Autodesk Inventor part; units mm, degrees
ref_plane "YZ Plane" through (0, 0, 0) normal (1, 0, 0) x (0, 1, 0)
ref_plane "XZ Plane" through (0, 0, 0) normal (0, 1, 0) x (-1, 0, 0)
ref_plane "XY Plane" through (0, 0, 0) normal (0, 0, 1) x (1, 0, 0)
sketch "Sketch1" plane through (0, 0, 0) normal (1, 0, 0) x (0, 1, 0)
  line L0 (0, 0) -> (25.4, 0)
  line L1 (25.4, 0) -> (25.4, -133.35)
  line L2 (25.4, -133.35) -> (0, -133.35)
  line L3 (0, -133.35) -> (0, 0)
  dimension "d0" = 25.4
  dimension "d1" = 133.35
extrude "Extrusion1" add sketch "Sketch1" along normal blind 6.35
sketch "Sketch2" plane through (6.35, 0, 0) normal (1, 0, 0) x (0, 0, -1)
  line L0 (133.35, 0) -> (133.35, 25.4)
  line L1 (133.35, 25.4) -> (0, 25.4)
  line L2 (0, 25.4) -> (0, 0)
  line L3 (0, 0) -> (133.35, 0)
  circle A0 centre (12.7, 12.7) radius 6.35
  circle A1 centre (120.65, 12.7) radius 6.35
  dimension "d4" = 25.4
  dimension "d5" = 12.7
  dimension "d6" = 12.7
  dimension "d7" = 107.95
  dimension "d8" = 133.35
  dimension "d9" = 12.7
  dimension "d10" = 12.7
  dimension "d11" = 12.7
extrude "Extrusion2" cut sketch "Sketch2" against normal blind 6.35 contours A0 | A1
sketch "Sketch3" plane through (6.35, 0, 0) normal (1, 0, 0) x (0, 0, -1)
  circle A0 centre (12.7, 12.7) radius 6.35
  circle A1 centre (12.7, 12.7) radius 12.7
  line L0 (133.35, 25.4) -> (0, 25.4)
  line L1 (0, 25.4) -> (0, 0)
  line L2 (0, 0) -> (133.35, 0)
  point P0 (12.7, 0)
  point P1 (0, 12.7)
  point P2 (12.7, 25.4)
extrude "Extrusion3" cut sketch "Sketch3" against normal blind 6.35 contours A1 L1 L0 | L2 L1 A1
sketch "Sketch4" plane through (6.35, 0, 0) normal (1, 0, 0) x (0, 0, -1)
  circle A0 centre (12.7, 12.7) radius 6.35
  line L0 (120.65, 12.7) -> (12.7, 12.7)
  circle A1 centre (120.65, 12.7) radius 6.35
  line L1 (12.7, 12.7) -> (120.65, -43.3755)
  line L2 (120.65, -43.3755) -> (120.65, 12.7)
  line L3 (12.7, 12.7) -> (9.1874, 5.9379)
  line L4 (9.1874, 5.9379) -> (43.1586, -11.7087)
  line L5 (43.1586, -11.7087) -> (46.6713, -4.9467)
  line L6 (12.7, 0) -> (133.35, 0)
  line L7 (46.6713, -4.9467) -> (49.2408, 0)
  point P0 (0, 0)
  point P1 (20.6183, 0)
  dimension "d16" = 27.45
  dimension "d19" = 25.4
  dimension "d22" = 7.62
extrude "Extrusion4" add sketch "Sketch4" against normal blind 6.35 contours L6 L7 L1 | L1 L5 L4 L6
properties part number "IntakeBraket"
Input: part model. Units: mm. Frame: model coordinates. A direction names the side the tool comes from. Give positions to 0.01 mm unless a question says otherwise; leave off trailing zeros. Write each loop counter-clockwise with the first axis right and the second up, starting at its lowest first coordinate (ties: lowest second). Pieces come first, ordered by that corner, then holes. Notation, with made-up numbers: (47.25, 61) - (71.25, 61) arc R13 cw to (71.25, 71) - close; hole circle Ø8 at (23.5, 72.5). An arc over 180 degrees is marked (long way). Write item = value, one per line. Start each with the question number.
1. Access query for faces 4 (the flat face through (3, 0, -92)), 5 (the cylindrical face through (3.22, 16.99, -8.02)), 6 (the flat face through (3, 0, -17)). Directions: +Z, -Z, +X, -X, +Y, -Y. A direction counts if a zero-diameter tool reaches every point of the face in a straight line with its end or side. Return the directions, or none.
2. Section query C-C, the plane z = -120.65. Output: boundary loops of the cut face in (x, y), then the cut area to 3 significant figures.
3. Section query B-B, the plane x = 2. Output: boundary loops of the cut face in (y, z), then the cut area to 3 significant figures.
4. Mould query, pull axis Z, two halves, no side actions, for faces 1 (the flat face through (0, 11, -66)), 2 (the cylindrical face through (3.219, 12.979, -0.003)), 3 (the cylindrical face through (3.219, 12.979, -114.306)). Classes: released by +Z, released by -Z, zero draft, split by the parting line, or undercut.
5. First-contact query: pin 1 Ø10 at (y, z) = (12.7, -12.7) entering from +X; pin 2 Ø1.5 at (x, y) = (1.5, -3.5) entering from +Z; pin 3 Ø2 at (x, y) = (4, -7.5) entering from -Z. Flat tips, straight axial feed; report the tip coordinate or a pass-through.
6. Section query A-A, the plane y = 12.7. Output: boundary loops of the cut face in (x, z), then the cut area to 3 significant figures.
7. Section query D-D, the plane y = 7.5. Output: boundary loops of the cut face in (x, z), then the cut area to 3 significant figures.
8. Ray query, L1, parallel to Z at x = 4.75, y = 7; L2, parallel to Y at x = 5, z = -12.7; L3, parallel to Z at x = 3.25, y = 9. Return the intervals inside material, ascending.
Check sheet entries:
q1.face_4 = -Z, +X, -X, -Y
q1.face_5 = +X, -X
q1.face_6 = +Z, +X, -X, -Y
q2.outline = (0, 0) - (6.35, 0) - (6.35, 6.35) - (0, 6.35) - close; (0, 19.05) - (6.35, 19.05) - (6.35, 25.4) - (0, 25.4) - close
q2.area = 80.6 mm2
q3.outline = (-11.71, -43.16) - (-4.95, -46.67) - (0, -49.24) - (0, -133.35) - (25.4, -133.35) - (25.4, -12.7) arc R12.7 ccw to (0, -12.7) - (0, -20.62) - close; hole circle Ø12.7 at (12.7, -120.65); hole circle Ø12.7 at (12.7, -12.7)
q3.area = 3,230 mm2
q4.face_1 = zero draft
q4.face_2 = released by +Z
q4.face_3 = undercut
q5.pin_1 = through
q5.pin_2 = -25.91
q5.pin_3 = -45.86
q6.outline = (0, -133.35) - (6.35, -133.35) - (6.35, -127) - (0, -127) - close; (0, -114.3) - (6.35, -114.3) - (6.35, -19.05) - (0, -19.05) - close; (0, -6.35) - (6.35, -6.35) - (6.35, 0) - (0, 0) - close
q6.area = 685 mm2
q7.outline = (0, -133.35) - (6.35, -133.35) - (6.35, -124.29) - (0, -124.29) - close; (0, -117.01) - (6.35, -117.01) - (6.35, -16.34) - (0, -16.34) - close; (0, -9.06) - (6.35, -9.06) - (6.35, -1.11) - (0, -1.11) - close
q7.area = 747 mm2
q8.L1 = -133.35 to -123.45, -117.85 to -15.5, -9.9 to -1.35
q8.L2 = 0 to 6.35, 19.05 to 25.4
q8.L3 = -133.35 to -125.81, -115.49 to -17.86, -7.54 to -0.55
